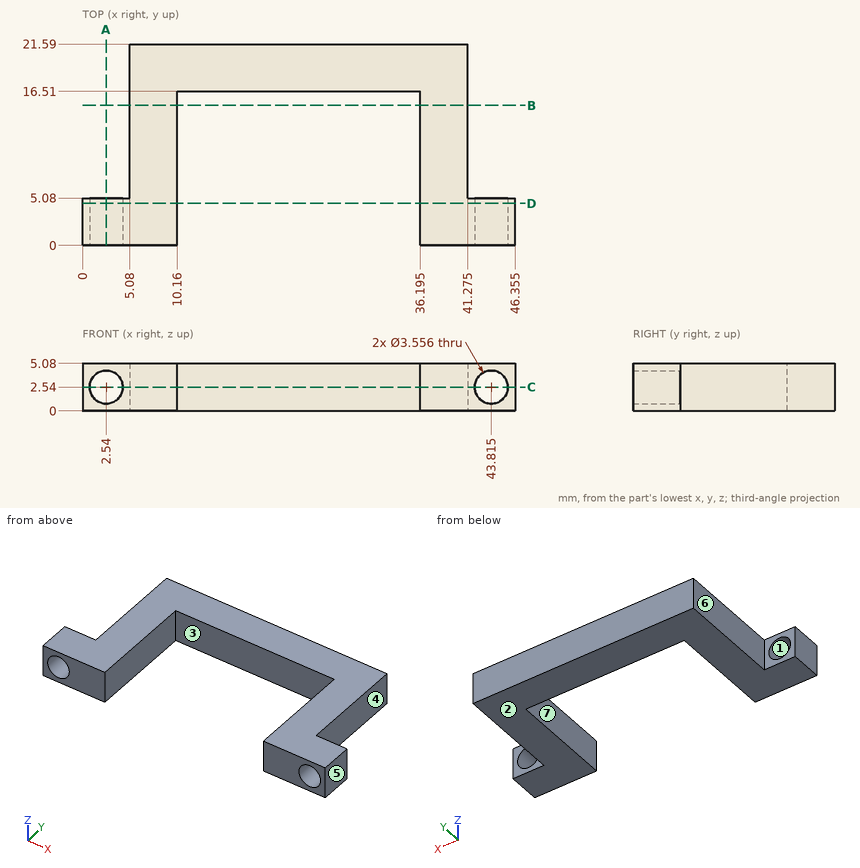
Study the drawing (mm; zero at the part's minimum x, y, z) and answer. A direction names the side the tool comes from. Coordinates: 2 decimals unless noted, no trailing zeros. Write each loop counter-clockwise with the first axis right and the second up, starting at its lowest first coordinate (ties: lowest second). Pieces come first, ordered by that corner, then holes.
Q1. A cutting plane is placed at D-D, the plane y = 4.5. Give the vertices of the cut face in (x, z) (3 decimals).
Q2. Each of these flat-tipped pins is pushed along its axis until it touches: pin 1 Ø3 at (x, z) = (43.815, 2.54) entering from -Y; pin 2 Ø2.5 at (y, z) = (11, 2) entering from -X; pin 3 Ø1.5 at (y, z) = (10, 2) entering from +X (3 decimals); pin 4 Ø1 at (x, z) = (22, 3) entering from -Y. Where does it stop, or does it pass through?
Q3. Find the intervals of material crossed by line 1 (X direction, y = 1.7, z = 2.54) (3 decimals); line 2 (X direction, y = 7, z = 1.95) (3 decimals); line 3 (X direction, y = 2.5, z = 1.6) (3 decimals), in increasing order.
Q4. A cutting plane is placed at A-A, the plane x = 2.54. Give the vertices of the cut face in (y, z), then the cut area to 3 significant figures.
Q5. Which of the six approach directions +Z, -Z, +X, -X, +Y, -Y give full straight-line access (tool end or side, diameter ignored) to the marked faces 4, 5, 6 and 7?
Q6. A cutting plane is placed at B-B, the plane y = 15. Give the vertices of the cut face in (x, z) (3 decimals).
Q7. A cutting plane is placed at C-C, the plane z = 2.54. Give the vertices of the cut face in (x, y) (3 decimals), then the cut area to 3 significant figures.
Q8. Determine the mould class of the marked faces 1, 2 and 3 for opening direction Z: released by +Z, released by -Z, zero draft, split by the parting line, or undercut.
Findings below:
1. outline: (0, 0) - (10.16, 0) - (10.16, 5.08) - (0, 5.08) - close; (36.195, 0) - (46.355, 0) - (46.355, 5.08) - (36.195, 5.08) - close; hole circle Ø3.556 at (2.54, 2.54); hole circle Ø3.556 at (43.815, 2.54)
2. pin 1: passes through
2. pin 2: stops at x = 5.08
2. pin 3: stops at x = 41.275
2. pin 4: stops at y = 16.51
3. line 1: x = 0 to 0.762, 4.318 to 10.16, 36.195 to 42.037, 45.593 to 46.355
3. line 2: x = 5.08 to 10.16, 36.195 to 41.275
3. line 3: x = 0 to 1.031, 4.049 to 10.16, 36.195 to 42.306, 45.324 to 46.355
4. outline: (0, 0) - (5.08, 0) - (5.08, 0.76) - (0, 0.76) - close; (0, 4.32) - (5.08, 4.32) - (5.08, 5.08) - (0, 5.08) - close
4. area: 7.74 mm2
5. face 4: +Z, -Z, +X, +Y
5. face 5: +Z, -Z, +X, +Y, -Y
5. face 6: +Z, -Z, -X, +Y
5. face 7: +Z, -Z, -Y
6. outline: (5.08, 0) - (10.16, 0) - (10.16, 5.08) - (5.08, 5.08) - close; (36.195, 0) - (41.275, 0) - (41.275, 5.08) - (36.195, 5.08) - close
7. outline: (0, 0) - (0.762, 0) - (0.762, 5.08) - (0, 5.08) - close; (4.318, 0) - (10.16, 0) - (10.16, 16.51) - (36.195, 16.51) - (36.195, 0) - (42.037, 0) - (42.037, 5.08) - (41.275, 5.08) - (41.275, 21.59) - (5.08, 21.59) - (5.08, 5.08) - (4.318, 5.08) - close; (45.593, 0) - (46.355, 0) - (46.355, 5.08) - (45.593, 5.08) - close
7. area: 367 mm2
8. face 1: undercut
8. face 2: released by -Z
8. face 3: zero draft
